Can you work these out from the model? Positions are in its coordinate system, mm. Round coordinates to 2 decimals unless told otherwise and drop trailing zeros. One line per item, written item: value. Start each with the question number.
(1) Thinking about a two-plate mould opening in Z: for faces 1 (the face through (-4.38, 19.11, 0.02)), 2 (the face through (-12.569, 16.824, 0.034)), 3 (the face through (-8.739, 20.075, 1.921)), which applies, +Z half, -Z half, draft (parallel to the pull), parting line (faces both ways), or undercut?
(2) I'm going to push flat-ended pins straight in: pin 1 Ø1 at (y, z) = (21, -2) entering from +X; pin 2 Ø2 at (x, z) = (-8.5, 1.5) entering from -Y; pin 3 Ø1 at (x, z) = (-8, -0.5) entering from -Y. Where does each tip first touch, or does it pass through?
(3) If I drill on L1, parallel to Z at x = -4, y = 16.5; L2, parallel to Z at x = -10.5, y = 20; L3, parallel to Y at x = -9.75, z = 2.3, over which ranges is the centre line in solid material (lowest first)? Write a range as from..to.
from build123d import *

# Parameters (mm, degrees)
ESQUISSE3_R             = 1.75
ENL_V_MAT_EXTRU_1_DEPTH = 0.5
ENL_V_MAT_EXTRU_1_DRAFT = -16
CONG_1_R                = 0.25


with BuildPart() as part:
    # Esquisse1 → Base-Révolution (revolve)
    with BuildSketch(Plane.XY, mode=Mode.PRIVATE) as base_r_volution_sk:
        Polygon((-3.894833669, 19.224673744), (-12.577919584, 16.857392814), (-13.2830375, 19.443735386), (-4.683927313, 22.119035716), align=None)
    revolve(base_r_volution_sk.sketch.rotate(Axis((3.55560583, 21.25589669, 0), (-0.9647873238288128, -0.2630312144579755, 0)), 180), axis=Axis((3.55560583, 21.25589669, 0), (-0.9647873238288128, -0.2630312144579755, 0)))


with BuildPart() as enl_v_mat_extru_1_tool:
    # Esquisse3 → Enlèv. mat.-Extru.1 (with draft: the straight prism first)
    with BuildSketch(Plane(origin=(1.253261753, 0.341678371, 0), x_dir=(0, 0, -1), z_dir=(0.9647873238288128, 0.26303121445797556, 0))):
        with Locations((0, 19.572184363)):
            Circle(ESQUISSE3_R)
    extrude(amount=-ENL_V_MAT_EXTRU_1_DEPTH)
    # Enlèv. mat.-Extru.1: the draft: its side faces are tilted about the plane it starts from
    enl_v_mat_extru_1_sides = [enl_v_mat_extru_1_tool.faces().sort_by_distance(p)[0] for p in [
        (-4.1360305, 19.158915941, 1.75),
    ]]
    draft(enl_v_mat_extru_1_sides, Plane(origin=(1.253261753, 0.341678371, 0), x_dir=(0, 0, -1), z_dir=(0.9647873238288128, 0.26303121445797556, 0)), ENL_V_MAT_EXTRU_1_DRAFT)


with BuildPart() as part_1:
    add(part.part)

    # Enlèv. mat.-Extru.1: cut by enl_v_mat_extru_1_tool
    add(enl_v_mat_extru_1_tool.part, mode=Mode.SUBTRACT)

    # Congé1
    cong_1_edges = [part_1.edges().sort_by_distance(p)[0] for p in [
        (-13.2830375, 19.443735386, 0),
        (-4.683927313, 22.119035716, 0),
    ]]
    fillet(cong_1_edges, radius=CONG_1_R)


solid = part_1.part
Established:
1. face 1: undercut
1. face 2: draft
1. face 3: parting line
2. pin 1: x = -4.24
2. pin 2: y = 15.01
2. pin 3: y = 15.09
3. L1: -1.44..1.44
3. L2: -1.25..1.25
3. L3: 16.03..19.28
